Geometry check sheet. Reference: drawing and pictorial views, mm from the part's lowest x, y, z. A direction names the side the tool comes from. Give positions to 0.01 mm unless a question says otherwise; leave off trailing zeros. Loops run counter-clockwise (first coordinate to the right, second up) from the corner with the lowest first, then second, coordinate; pieces in that order, holes last. Notation, with made-up numbers: (64, 75) - (93, 75) arc R32 ccw to (93, 107) - close; hole circle Ø2 at (65.25, 35). An arc over 180 degrees is marked (long way). Answer in a Markdown table with one row per item. Add a question column.
(1) Sectioned sample at B-B on y = 3.5. Enter the section's corners in (x, z), then the cut area to 3 significant figures.
(2) Sectioned sample at C-C on x = 5.75. Enter the section's corners in (y, z), then the cut area to 3 significant figures.
(3) Go/stop test with flat-tipped pins: P1, Ø1, axis at x = 7, z = 6.5, coming from the +Y side; P2, Ø1.3, axis at x = 4, y = 12, coming from the +Z side; P3, Ø1, axis at y = 10.5, z = 4, coming from the +X side. Record where each tip stops, or that it passes through.
(4) Sectioned sample at A-A on z = 8.5. Enter the section's corners in (x, y).
(5) Draft check along Z on the marked faces 5, 6 and 7. Enter one of: released by +Z, released by -Z, zero draft, split by the parting line, or undercut.
(6) Thickness scan on L1, parallel to Y at x = 4, z = 4.75; L2, parallel to Z at x = 8.5, y = 4.25. Record the ranges inside material, lowest first.
(7) Sectioned sample at D-D on z = 5. Enter the section's corners in (x, y).
(8) Set-up check for the marked faces 1, 2, 3 and 4: record each of +Z, -Z, +X, -X, +Y, -Y from which the full face is reachable in a straight line by a thin tool's end or side.
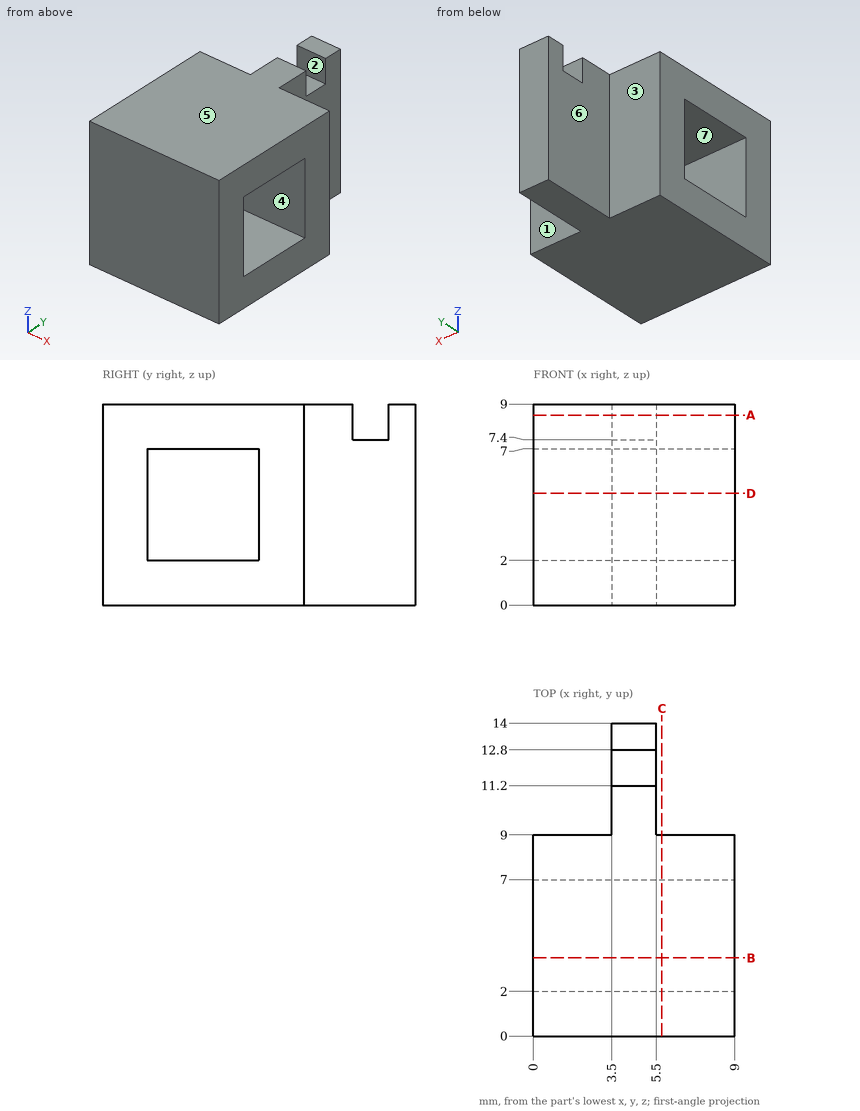
Reply:
| question | item | result |
|---|---|---|
| 1 | outline | (0, 0) - (9, 0) - (9, 2) - (0, 2) - close; (0, 7) - (9, 7) - (9, 9) - (0, 9) - close |
| 1 | area | 36.0 mm^2 |
| 2 | outline | (0, 0) - (9, 0) - (9, 9) - (0, 9) - close; hole (2, 2) - (7, 2) - (7, 7) - (2, 7) - close |
| 2 | area | 56.0 mm^2 |
| 3 | P1 | y = 9 |
| 3 | P2 | z = 7.4 |
| 3 | P3 | x = 5.5 |
| 4 | outline | (0, 0) - (9, 0) - (9, 9) - (5.5, 9) - (5.5, 11.2) - (3.5, 11.2) - (3.5, 9) - (0, 9) - close; (3.5, 12.8) - (5.5, 12.8) - (5.5, 14) - (3.5, 14) - close |
| 5 | face 5 | released by +Z |
| 5 | face 6 | zero draft |
| 5 | face 7 | undercut |
| 6 | L1 | 0 to 2, 7 to 14 |
| 6 | L2 | 0 to 2, 7 to 9 |
| 7 | outline | (0, 0) - (9, 0) - (9, 2) - (0, 2) - close; (0, 7) - (9, 7) - (9, 9) - (5.5, 9) - (5.5, 14) - (3.5, 14) - (3.5, 9) - (0, 9) - close |
| 8 | face 1 | +Z, -Z, +X, +Y |
| 8 | face 2 | +Z, +X, -X |
| 8 | face 3 | +Z, -Z, -X, +Y |
| 8 | face 4 | +X, -X |
